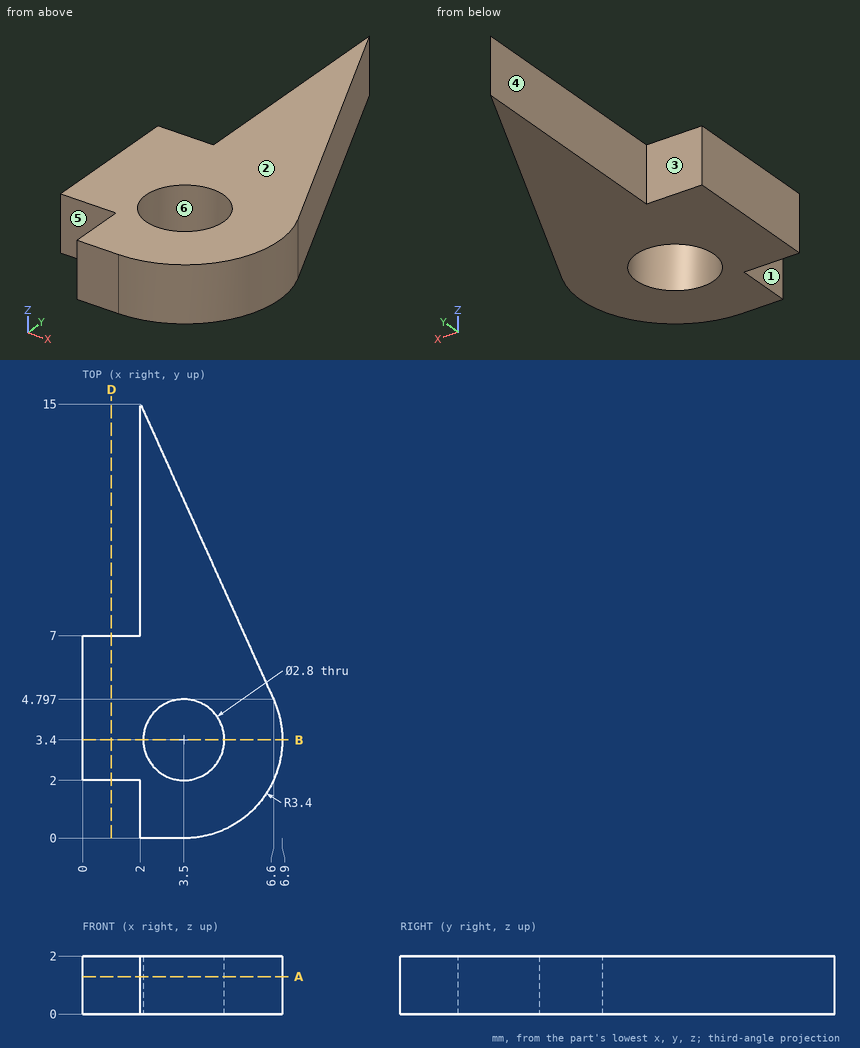
Source: three-view drawing plus pictorial views. Frame: mm from the lowest corner of the part. A direction names the side the tool comes from. Coordinates: 2 decimals unless noted, no trailing zeros. Order: outer loops, then holes, each group sorted by start corner. A loop starts at its lowest first (then second) coordinate and runs counter-clockwise, first axis right, second up. Notation, with made-up numbers: M 77.25,-10.75 L 125.25,-10.75 A20 cw 125.25,-2.75 Z; hole C 27.5,37.5 d7. An arc over 180 degrees is marked long. One line per question, with ' | ' between items. Start each with the question number.
Item 1: Pin query (flat end, axial travel): pin 1 Ø1 at (y, z) = (10, 0.5) entering from -X. Return the tip coordinate at first contact, or that it passes through.
Item 2: Draft query along Y for the marked faces 4, 5 and 6. Return one class per face: released by +Y, released by -Y, zero draft, split by the parting line, or undercut.
Item 3: Cut plane D-D, the plane x = 1. Return the cut outline in (y, z), then the cut area to 3 significant figures.
Item 4: Ray query, probe 1 along Y at (x, z) = (3.5, 0.9) (1 decimal); probe 2 along X at (y, z) = (4.5, 1.55) (1 decimal); probe 3 along Y at (x, z) = (2.5, 0.45) (1 decimal). Return the intervals inside material, ascending. Write a range as [from, to].
Item 5: Cut plane A-A, the plane z = 1.3. Return the cut outline in (x, y), then the cut area to 3 significant figures.
Item 6: Set-up query: the marked faces 1, 2 and 3. Return all of +Z, -Z, +X, -X, +Y, -Y with unobstructed straight access to the full face (end or side cutting, diameter ignored); none if empty.
Item 7: Cut plane B-B, the plane y = 3.4. Return the cut outline in (x, z).
A:
1) pin 1: stops at x = 2
2) face 4: zero draft | face 5: released by -Y | face 6: undercut
3) outline: M 2,0 L 7,0 L 7,2 L 2,2 Z | area: 10.0 mm2
4) probe 1: y = [0, 2], [4.8, 11.7] | probe 2: x = [0, 2.6], [4.4, 6.7] | probe 3: y = [0, 2.4], [4.4, 13.9]
5) outline: M 0,2 L 2,2 L 2,0 L 3.5,0 A3.4 ccw 6.6,4.8 L 2,15 L 2,7 L 0,7 Z; hole C 3.5,3.4 d2.8 | area: 48.2 mm2
6) face 1: +Z, -Z, -X, -Y | face 2: +Z, +X, -X, +Y, -Y | face 3: +Z, -Z, -X, +Y
7) outline: M 0,0 L 2.1,0 L 2.1,2 L 0,2 Z; M 4.9,0 L 6.9,0 L 6.9,2 L 4.9,2 Z
